Check sheet for the modelled part. Datum: model origin and axes. Units: mm. A direction names the side the tool comes from. Coordinates: 2 decimals unless noted, no trailing zeros. Write each loop counter-clockwise with the first axis right and the second up, starting at its lowest first coordinate (ties: lowest second). Pieces come first, ordered by that corner, then holes. Notation, with made-up numbers: M -2.75,73.25 L 6.25,73.25 A25 ccw 6.25,110.25 Z; hole C -25,-28.75 d2. An arc over 180 degrees is marked long. Answer as CSV lines item,"result". Start each with the question number.
Q1. Thickness scan on line 1 along Z through (x, y) = (40, 22.5); line 2 along Y through (x, z) = (44.5, -43.5); line 3 along Y through (x, z) = (43.25, -23.5). Record the ranges inside material, lowest first. Write a range as from..to.
Q2. Sectioned sample at B-B, the plane y = 15.5. Record the cut outline in (x, z), then the cut area to 3 significant figures.
Q3. Sectioned sample at A-A, the plane z = -11. Record the cut outline in (x, y).
Q4. Depth check by flat-ended pin: pin 1 Ø1.5 at (x, y) = (38.5, -11.5) entering from +Z; pin 2 Ø0.8 at (y, z) = (-21.5, -28) entering from +X; pin 3 Ø2 at (y, z) = (15.5, -43.5) entering from +X. Enter the tip coordinate at first touch or a pass-through.
Q5. Access from +Z, -Z, +X, -X, +Y, -Y to the whole of each face (thin tool, end or side, straight path). Record for faces 4 (the flat face through (37, -17.254, -27)), 5 (the flat face through (42, -6, 2)), 6 (the cylindrical face through (43.065, -24.334, -26.261)).
Q6. Mould release check, pull along Z, two halves, no side actions. Record for faces 1 (the flat face through (43, -27.566, -11)), 2 (the cylindrical face through (43.241, 25.578, 2.098)), 3 (the flat face through (40.565, -6, 1)): pulls with the +Z half, pulls with the -Z half, needs draft (parallel to the pull), parting line crosses it, or undercut.
from build123d import *

# Parameters (mm, degrees)
CROQUIS1_W                   = 3.246579248
CROQUIS1_H                   = 8.852829877
SALIENTE_EXTRUIR1_DEPTH      = 2
CROQUIS5_W                   = 9
CROQUIS5_H                   = 0.5
ARREGLO_IMPRESION1_DEPTH     = 2
CROQUIS6_W                   = 9
CROQUIS6_H                   = 48
SALIENTE_EXTRUIR4_DEPTH      = 2
CROQUIS7_W                   = 9
CROQUIS7_H                   = 48
SALIENTE_EXTRUIR5_DEPTH      = 2
CROQUIS8_W                   = 9
CROQUIS8_H                   = 50
SALIENTE_EXTRUIR6_DEPTH      = 2
SALIENTE_EXTRUIR7_DEPTH      = 1.7
SALIENTE_EXTRUIR7_DEPTH_BACK = 0.3
CROQUIS9_W                   = 50
CROQUIS9_H                   = 50
CROQUIS10_W                  = 10
CROQUIS10_H                  = 0.5
CORTAR_EXTRUIR1_DEPTH        = 8.700001
CROQUIS11_W                  = 3.246579248
CROQUIS11_H                  = 8.852829877
SALIENTE_EXTRUIR8_DEPTH      = 1
CROQUIS12_W                  = 10.7
CROQUIS12_H                  = 51
SALIENTE_EXTRUIR9_DEPTH      = 2
CROQUIS13_W                  = 10.7
CROQUIS13_H                  = 52
SALIENTE_EXTRUIR10_DEPTH     = 1
CROQUIS14_W                  = 10.7
CROQUIS14_H                  = 52
SALIENTE_EXTRUIR11_DEPTH     = 2
SALIENTE_EXTRUIR12_DEPTH     = 6.5
CORTAR_EXTRUIR2_START        = -7
CROQUIS19_R                  = 1.625
CORTAR_EXTRUIR2_DEPTH        = 7
CORTAR_EXTRUIR3_DEPTH        = 2.5
CROQUIS22_W                  = 10
CROQUIS22_H                  = 2
CORTAR_EXTRUIR4_DEPTH        = 8.7
CORTAR_EXTRUIR5_START        = -10.7
CORTAR_EXTRUIR5_DEPTH        = 10.7
REDONDEO4_R                  = 3
CROQUIS24_W                  = 5.246579248
CROQUIS24_H                  = 10.87000641
CORTAR_EXTRUIR6_DEPTH        = 3
CORTAR_EXTRUIR6_DRAFT        = -18
CROQUIS25_W                  = 6.58
CROQUIS25_H                  = 11.7
CORTAR_EXTRUIR7_DEPTH        = 2


with BuildPart() as part:
    # Croquis1 → Saliente-Extruir1 (new body)
    with BuildSketch(Plane.XY):
        Polygon((47.144751496, 21.933935563), (38.144751496, 21.933935563), (38.144751496, -23.066064437), (47.144751496, -23.066064437), (47.144751496, -9.741064437), (42.564751496, -9.741064437), (42.564751496, -2.041064437), (47.144751496, -2.041064437), align=None)
        with Locations((43.941461872, -18.353940173)):
            Rectangle(CROQUIS1_W, CROQUIS1_H, mode=Mode.SUBTRACT)
    extrude(amount=SALIENTE_EXTRUIR1_DEPTH)

    # Croquis5 → Arreglo_impresion1 (add)
    with BuildSketch(Plane.XY.offset(2)):
        with Locations((42.644751496, -23.316064437)):
            Rectangle(CROQUIS5_W, CROQUIS5_H)
        with Locations((42.644751496, 22.183935563)):
            Rectangle(CROQUIS5_W, CROQUIS5_H)
    extrude(amount=-ARREGLO_IMPRESION1_DEPTH)

    # Croquis6 → Saliente-Extruir4 (add)
    with BuildSketch(Plane.XZ.offset(23.566064437)):
        with Locations((42.644751496, -22)):
            Rectangle(CROQUIS6_W, CROQUIS6_H)
    extrude(amount=SALIENTE_EXTRUIR4_DEPTH)

    # Croquis7 → Saliente-Extruir5 (add)
    with BuildSketch(Plane(origin=(0, 0, -46), x_dir=(-1, 0, 0), z_dir=(0, 0, -1))):
        with Locations((-42.644751496, -1.566064437)):
            Rectangle(CROQUIS7_W, CROQUIS7_H)
    extrude(amount=SALIENTE_EXTRUIR5_DEPTH)

    # Croquis8 → Saliente-Extruir6 (add)
    with BuildSketch(Plane(origin=(0, 22.433935563, 0), x_dir=(1, 0, 0), z_dir=(0, 1, 0))):
        with Locations((42.644751496, 23)):
            Rectangle(CROQUIS8_W, CROQUIS8_H)
    extrude(amount=SALIENTE_EXTRUIR6_DEPTH)

    # Croquis9 → Saliente-Extruir7 (add, two sides: drawn at the far end of the back side and taken through both)
    with BuildSketch(Plane.ZY.offset(-38.144751496).offset(-SALIENTE_EXTRUIR7_DEPTH_BACK)):
        with Locations((-23, -0.566064437)):
            Rectangle(CROQUIS9_W, CROQUIS9_H)
        with BuildLine():
            Line((-29.385, -14.254496437), (-24.885, -14.254496437))
            ThreePointArc((-24.885, -14.254496437), (-23.885, -15.254496437), (-24.885, -16.254496437))
            Line((-24.885, -16.254496437), (-29.385, -16.254496437))
            ThreePointArc((-29.385, -16.254496437), (-30.385, -15.254496437), (-29.385, -14.254496437))
        make_face(mode=Mode.SUBTRACT)
        with BuildLine():
            Line((-29.385, -17.254496437), (-24.885, -17.254496437))
            ThreePointArc((-24.885, -17.254496437), (-23.885, -18.254496437), (-24.885, -19.254496437))
            Line((-24.885, -19.254496437), (-29.385, -19.254496437))
            ThreePointArc((-29.385, -19.254496437), (-30.385, -18.254496437), (-29.385, -17.254496437))
        make_face(mode=Mode.SUBTRACT)
    extrude(amount=SALIENTE_EXTRUIR7_DEPTH + SALIENTE_EXTRUIR7_DEPTH_BACK)

    # Croquis10 → Cortar-Extruir1 (cut)
    with BuildSketch(Plane(origin=(47.144751496, 0, 0), x_dir=(0, 0, -1), z_dir=(1, 0, 0))):
        with Locations((33.991483973, 22.683935563)):
            Rectangle(CROQUIS10_W, CROQUIS10_H)
    extrude(amount=-CORTAR_EXTRUIR1_DEPTH, mode=Mode.SUBTRACT)

    # Croquis11 → Saliente-Extruir8 (add)
    with BuildSketch(Plane.XY.offset(2)):
        Polygon((47.144751496, 24.433935563), (36.444751496, 24.433935563), (36.444751496, -25.566064437), (47.144751496, -25.566064437), (47.144751496, -9.741064437), (42.564751496, -9.741064437), (42.564751496, -2.041064437), (47.144751496, -2.041064437), align=None)
        with Locations((43.941461872, -18.353940173)):
            Rectangle(CROQUIS11_W, CROQUIS11_H, mode=Mode.SUBTRACT)
    extrude(amount=SALIENTE_EXTRUIR8_DEPTH)

    # Croquis12 → Saliente-Extruir9 (add)
    with BuildSketch(Plane.XZ.offset(25.566064437)):
        with Locations((41.794751496, -22.5)):
            Rectangle(CROQUIS12_W, CROQUIS12_H)
    extrude(amount=SALIENTE_EXTRUIR9_DEPTH)

    # Croquis13 → Saliente-Extruir10 (add)
    with BuildSketch(Plane(origin=(0, 0, -48), x_dir=(-1, 0, 0), z_dir=(0, 0, -1))):
        with Locations((-41.794751496, -1.566064437)):
            Rectangle(CROQUIS13_W, CROQUIS13_H)
    extrude(amount=SALIENTE_EXTRUIR10_DEPTH)

    # Croquis14 → Saliente-Extruir11 (add)
    with BuildSketch(Plane(origin=(0, 24.433935563, 0), x_dir=(1, 0, 0), z_dir=(0, 1, 0))):
        with Locations((41.794751496, 23)):
            Rectangle(CROQUIS14_W, CROQUIS14_H)
    extrude(amount=SALIENTE_EXTRUIR11_DEPTH)

    # Croquis17 → Saliente-Extruir12 (add)
    with BuildSketch(Plane(origin=(38.444751496, 0, 0), x_dir=(0, 0, -1), z_dir=(1, 0, 0))):
        Polygon((22.135, -20.566064437), (32.135, -20.566064437), (35.135, -23.566064437), (19.135, -23.566064437), align=None)
    extrude(amount=SALIENTE_EXTRUIR12_DEPTH)

    # Croquis19 → Cortar-Extruir2 (cut)
    with BuildSketch(Plane(origin=(0, -20.566064437, 0), x_dir=(1, 0, 0), z_dir=(0, 1, 0)).offset(CORTAR_EXTRUIR2_START)):
        with Locations(Location((41.694751496, 27.135, 0), (0, 0, 270))):
            Circle(CROQUIS19_R)
    extrude(amount=CORTAR_EXTRUIR2_DEPTH, mode=Mode.SUBTRACT)

    # Croquis20 → Cortar-Extruir3 (cut)
    with BuildSketch(Plane(origin=(0, -20.566064437, 0), x_dir=(1, 0, 0), z_dir=(0, 1, 0))):
        Polygon((41.694751496, 30.335), (38.923470204, 28.735), (38.923470204, 25.535), (41.694751496, 23.935), (44.466032788, 25.535), (44.466032788, 28.735), align=None)
    extrude(amount=-CORTAR_EXTRUIR3_DEPTH, mode=Mode.SUBTRACT)

    # Croquis22 → Cortar-Extruir4 (cut)
    with BuildSketch(Plane(origin=(47.144751496, 0, 0), x_dir=(0, 0, -1), z_dir=(1, 0, 0))):
        with Locations((27.135, -26.566064437)):
            Rectangle(CROQUIS22_W, CROQUIS22_H)
        with Locations((9.331412976, 23.433935563)):
            Rectangle(CROQUIS22_W, CROQUIS22_H)
    extrude(amount=-CORTAR_EXTRUIR4_DEPTH, mode=Mode.SUBTRACT)

    # Croquis23 → Cortar-Extruir5 (cut)
    with BuildSketch(Plane(origin=(47.144751496, 0, 0), x_dir=(0, 0, -1), z_dir=(1, 0, 0)).offset(CORTAR_EXTRUIR5_START)):
        with BuildLine():
            Line((-3, -27.566064437), (0, -27.566064437))
            ThreePointArc((0, -27.566064437), (-2.121320344, -26.687384781), (-3, -24.566064437))
            Line((-3, -24.566064437), (-3, -27.566064437))
        make_face()
        with BuildLine():
            Line((-3, 26.433935563), (0, 26.433935563))
            ThreePointArc((0, 26.433935563), (-2.121320344, 25.555255907), (-3, 23.433935563))
            Line((-3, 23.433935563), (-3, 26.433935563))
        make_face()
        with BuildLine():
            Line((49, 26.433935563), (49, 23.433935563))
            ThreePointArc((49, 23.433935563), (48.121320344, 25.555255907), (46, 26.433935563))
            Line((46, 26.433935563), (49, 26.433935563))
        make_face()
        with BuildLine():
            Line((49, -27.566064437), (46, -27.566064437))
            ThreePointArc((46, -27.566064437), (48.121320344, -26.687384781), (49, -24.566064437))
            Line((49, -24.566064437), (49, -27.566064437))
        make_face()
    extrude(amount=CORTAR_EXTRUIR5_DEPTH, mode=Mode.SUBTRACT)

    # Redondeo4
    # the kernel refuses this fillet: 3 mm, written as the material it takes off along each edge
    with BuildSketch(Plane(origin=(36.444751496, -24.566064437, 0), x_dir=(0, -1, 0), z_dir=(0, 0, -1))) as redondeo4_piece_1:
        with BuildLine():
            CenterArc((3 - REDONDEO4_R, -REDONDEO4_R), REDONDEO4_R, 360, 90)
            Line((3, -REDONDEO4_R), (3, 0))
            Line((3, 0), (3 - REDONDEO4_R, 0))
        make_face()
    revolve(axis=Axis((36.444751496, -24.566064437, 0), (-1, 0, 0)), revolution_arc=90, mode=Mode.SUBTRACT)
    with BuildSketch(Plane(origin=(36.444751496, -24.566064437, 3), x_dir=(0, 0, -1), z_dir=(0, 1, 0)), Plane(origin=(36.444751496, 23.433935563, -49), x_dir=(0, 0, 1), z_dir=(0, -1, 0))) as redondeo4_piece_2:
        with BuildLine():
            CenterArc((REDONDEO4_R, -REDONDEO4_R), REDONDEO4_R, 90, 90)
            Line((0, -REDONDEO4_R), (0, 0))
            Line((0, 0), (REDONDEO4_R, 0))
        make_face()
    extrude(amount=48, mode=Mode.SUBTRACT)
    with BuildSketch(Plane(origin=(36.444751496, 23.433935563, 0), x_dir=(0, 1, 0), z_dir=(0, 0, -1))) as redondeo4_piece_3:
        with BuildLine():
            CenterArc((3 - REDONDEO4_R, REDONDEO4_R), REDONDEO4_R, 270, 90)
            Line((3, REDONDEO4_R), (3, 0))
            Line((3, 0), (3 - REDONDEO4_R, 0))
        make_face()
    revolve(axis=Axis((36.444751496, 23.433935563, 0), (1, 0, 0)), revolution_arc=90, mode=Mode.SUBTRACT)
    with BuildSketch(Plane(origin=(36.444751496, 26.433935563, -46), x_dir=(0, -1, 0), z_dir=(0, 0, 1))) as redondeo4_piece_4:
        with BuildLine():
            CenterArc((REDONDEO4_R, REDONDEO4_R), REDONDEO4_R, 180, 90)
            Line((0, REDONDEO4_R), (0, 0))
            Line((0, 0), (REDONDEO4_R, 0))
        make_face()
    extrude(amount=46, mode=Mode.SUBTRACT)
    with BuildSketch(Plane(origin=(36.444751496, 23.433935563, -46), x_dir=(0, 0, -1), z_dir=(0, -1, 0))) as redondeo4_piece_5:
        with BuildLine():
            CenterArc((3 - REDONDEO4_R, REDONDEO4_R), REDONDEO4_R, 270, 90)
            Line((3, REDONDEO4_R), (3, 0))
            Line((3, 0), (3 - REDONDEO4_R, 0))
        make_face()
    revolve(axis=Axis((36.444751496, 23.433935563, -46), (1, 0, 0)), revolution_arc=90, mode=Mode.SUBTRACT)
    with BuildSketch(Plane(origin=(36.444751496, -24.566064437, -46), x_dir=(0, -1, 0), z_dir=(0, 0, 1))) as redondeo4_piece_6:
        with BuildLine():
            CenterArc((3 - REDONDEO4_R, REDONDEO4_R), REDONDEO4_R, 270, 90)
            Line((3, REDONDEO4_R), (3, 0))
            Line((3, 0), (3 - REDONDEO4_R, 0))
        make_face()
    revolve(axis=Axis((36.444751496, -24.566064437, -46), (1, 0, 0)), revolution_arc=90, mode=Mode.SUBTRACT)
    with BuildSketch(Plane(origin=(36.444751496, -27.566064437, -46), x_dir=(0, 1, 0), z_dir=(0, 0, 1))) as redondeo4_piece_7:
        with BuildLine():
            CenterArc((REDONDEO4_R, -REDONDEO4_R), REDONDEO4_R, 90, 90)
            Line((0, -REDONDEO4_R), (0, 0))
            Line((0, 0), (REDONDEO4_R, 0))
        make_face()
    extrude(amount=46, mode=Mode.SUBTRACT)


with BuildPart() as cortar_extruir6_tool:
    # Croquis24 → Cortar-Extruir6 (with draft: the straight prism first)
    with BuildSketch(Plane.XY.offset(3)):
        with Locations((43.941461872, -18.36252844)):
            Rectangle(CROQUIS24_W, CROQUIS24_H)
    extrude(amount=-CORTAR_EXTRUIR6_DEPTH)
    # Cortar-Extruir6: the draft: its side faces are tilted about the plane it starts from
    cortar_extruir6_sides = [cortar_extruir6_tool.faces().sort_by_distance(p)[0] for p in [
        (43.941461872, -23.797531645, 1.5),
        (46.564751496, -18.36252844, 1.5),
        (43.941461872, -12.927525235, 1.5),
        (41.318172248, -18.36252844, 1.5),
    ]]
    draft(cortar_extruir6_sides, Plane.XY.offset(3), CORTAR_EXTRUIR6_DRAFT)


with BuildPart() as part_1:
    add(part.part)

    # Cortar-Extruir6: cut by cortar_extruir6_tool
    add(cortar_extruir6_tool.part, mode=Mode.SUBTRACT)

    # Croquis25 → Cortar-Extruir7 (cut)
    with BuildSketch(Plane(origin=(0, 0, 0), x_dir=(-1, 0, 0), z_dir=(0, 0, -1))):
        with Locations((-43.854751496, -5.891064437)):
            Rectangle(CROQUIS25_W, CROQUIS25_H)
    extrude(amount=-CORTAR_EXTRUIR7_DEPTH, mode=Mode.SUBTRACT)


solid = part_1.part
Output:
1,line 1,"z = -49..-38.99, -28.99..-14.33, -4.33..3"
1,line 2,"y = -27.57..-23.57, 22.43..26.43"
1,line 3,"y = -25.57..-20.57, 22.43..26.43"
2,outline,"M 36.44,-46 A3 ccw 39.44,-49 L 47.14,-49 L 47.14,-46 L 38.44,-46 L 38.44,0 L 47.14,0 L 47.14,3 L 39.44,3 A3 ccw 36.44,0 Z"
2,area,"152 mm^2"
3,outline,"M 36.44,-24.57 A3 ccw 39.44,-27.57 L 47.14,-27.57 L 47.14,-23.57 L 38.44,-23.57 L 38.44,24.43 L 47.14,24.43 L 47.14,26.43 L 39.44,26.43 A3 ccw 36.44,23.43 Z"
4,pin 1,"stops at z = 2.99"
4,pin 2,"stops at x = 44.94"
4,pin 3,"stops at x = 38.44"
5,face 4,"+X, -X"
5,face 5,"+X"
5,face 6,"-Y"
6,face 1,"needs draft"
6,face 2,"pulls with the +Z half"
6,face 3,"undercut"
